from build123d import *

# Parameters (mm, degrees)
SKETCH1_W               = 134.83
SKETCH1_H               = 45.93
SKETCH1_W_2             = 124.83
SKETCH1_H_2             = 35.93
BOSS_EXTRUDE1_DEPTH     = 2.5
BOSS_EXTRUDE2_START     = 2.5
SKETCH1_3_W             = 134.83
SKETCH1_3_H             = 45.93
SKETCH1_3_W_2           = 124.83
SKETCH1_3_H_2           = 35.93
BOSS_EXTRUDE2_DEPTH     = 2.5
SKETCH2_R               = 6.25
SKETCH2_R_2             = 3.25
BOSS_EXTRUDE3_DEPTH     = 5
FILLET1_R               = 10
CUT_EXTRUDE4_DEPTH      = 78.396792246
CUT_EXTRUDE4_DEPTH_BACK = 78.396792246
SKETCH5_W               = 10
SKETCH5_H               = 5
SKETCH6_R               = 1
CUT_EXTRUDE5_DEPTH      = 4
SKETCH7_W               = 7
SKETCH7_H               = 25.4
SKETCH7_W_2             = 8
BOSS_EXTRUDE4_DEPTH     = 7.5
BOSS_EXTRUDE5_START     = -7.5
SKETCH7_4_W             = 8
SKETCH7_4_H             = 25.4
BOSS_EXTRUDE5_DEPTH     = 25.4


with BuildPart() as part:
    # Sketch1 → Boss-Extrude1 (new, symmetric)
    # profile 1 of 2: a face of its own
    with BuildSketch(Plane.XY):
        Rectangle(SKETCH1_W, SKETCH1_H)
        Rectangle(SKETCH1_W_2, SKETCH1_H_2, mode=Mode.SUBTRACT)
    # profile 2 of 2: a face of its own
    with BuildSketch(Plane.XY):
        Rectangle(SKETCH1_W_2, SKETCH1_H_2)
    extrude(amount=BOSS_EXTRUDE1_DEPTH, both=True)

    # Sketch1<3> → Boss-Extrude2 (add, symmetric)
    with BuildSketch(Plane.XY.offset(BOSS_EXTRUDE2_START)):
        Rectangle(SKETCH1_3_W, SKETCH1_3_H)
        Rectangle(SKETCH1_3_W_2, SKETCH1_3_H_2, mode=Mode.SUBTRACT)
    extrude(amount=BOSS_EXTRUDE2_DEPTH, both=True)

    # Sketch2 → Boss-Extrude3 (add)
    # profile 1 of 2: a face of its own
    with BuildSketch(Plane.XZ.offset(22.965)):
        with BuildLine():
            ThreePointArc((6.25, 21.55), (-1.088960505, 15.395597915), (-5.870532806, 23.694608256))
            Line((-5.870532806, 23.694608256), (-12.7, 5))
            Line((-12.7, 5), (12.7, 5))
            Line((12.7, 5), (5.870532806, 23.694608256))
            ThreePointArc((5.870532806, 23.694608256), (6.154402085, 22.638960505), (6.25, 21.55))
        make_face()
    # profile 2 of 2: a face of its own
    with BuildSketch(Plane.XZ.offset(22.965)):
        with Locations((0, 21.55)):
            Circle(SKETCH2_R)
        with Locations(Location((0, 21.55, 0), (0, 0, 270))):
            Circle(SKETCH2_R_2, mode=Mode.SUBTRACT)
    extrude(amount=-BOSS_EXTRUDE3_DEPTH)

    # Fillet1
    fillet1_edges = [part.edges().sort_by_distance(p)[0] for p in [
        (-12.7, -20.465, 5),
        (12.7, -20.465, 5),
    ]]
    fillet(fillet1_edges, radius=FILLET1_R)

    # Sketch5 → Cut-Extrude4 (cut, two sides: drawn at the far end of the back side and taken through both)
    with BuildSketch(Plane(origin=(0, 0, -2.5), x_dir=(-1, 0, 0), z_dir=(0, 0, -1)).offset(-CUT_EXTRUDE4_DEPTH_BACK)):
        with Locations((7, 10.465)):
            Rectangle(SKETCH5_W, SKETCH5_H)
        with Locations((-7, 10.465)):
            Rectangle(SKETCH5_W, SKETCH5_H)
    extrude(amount=CUT_EXTRUDE4_DEPTH + CUT_EXTRUDE4_DEPTH_BACK, mode=Mode.SUBTRACT)

    # Sketch6 → Cut-Extrude5 (cut)
    with BuildSketch(Plane.ZY.offset(2)):
        with Locations((0, 10.465)):
            Circle(SKETCH6_R)
    extrude(amount=-CUT_EXTRUDE5_DEPTH, mode=Mode.SUBTRACT)

    # Sketch7 → Boss-Extrude4 (add)
    with BuildSketch(Plane(origin=(0, 0, -2.5), x_dir=(-1, 0, 0), z_dir=(0, 0, -1))):
        with Locations((-70.915, 0)):
            Rectangle(SKETCH7_W, SKETCH7_H)
        with Locations((-78.415, 0)):
            Rectangle(SKETCH7_W_2, SKETCH7_H)
        with Locations((78.415, 0)):
            Rectangle(SKETCH7_W_2, SKETCH7_H)
        with Locations((70.915, 0)):
            Rectangle(SKETCH7_W, SKETCH7_H)
    extrude(amount=-BOSS_EXTRUDE4_DEPTH)

    # Sketch7<4> → Boss-Extrude5 (add)
    with BuildSketch(Plane(origin=(0, 0, -2.5), x_dir=(-1, 0, 0), z_dir=(0, 0, -1)).offset(BOSS_EXTRUDE5_START)):
        with Locations((-78.415, 0)):
            Rectangle(SKETCH7_4_W, SKETCH7_4_H)
        with Locations((78.415, 0)):
            Rectangle(SKETCH7_4_W, SKETCH7_4_H)
    extrude(amount=-BOSS_EXTRUDE5_DEPTH)


solid = part.part
Work out the finished part from the listing and answer in its coordinate system (mm). A direction names the side the tool comes from. Give positions to 0.01 mm unless a question says otherwise; leave off trailing zeros. Order: outer loops, then holes, each group sorted by start corner. A loop starts at its lowest first (then second) coordinate and runs counter-clockwise, first axis right, second up. Notation, with made-up numbers: M 40.25,-14 L 54.25,-14 A13 ccw 54.25,7 Z; hole C 61,-29.75 d4. An arc over 180 degrees is marked long. Return JSON: item names as keys, results as strings.
Q1. The mould has two halves that part along X. Classify faces 1 (the face through (-77, 12.7, 10)), 2 (the face through (-1, 0, 2.5)), 3 (the face through (8.116, -20.5, 17.547)), 4 (the face through (-67.415, -18, 1)): pulls with the +X half, pulls with the -X half, needs draft (parallel to the pull), parting line crosses it, or undercut.
Answer below:
{"face 1": "needs draft", "face 2": "undercut", "face 3": "pulls with the +X half", "face 4": "pulls with the -X half"}
Q2. Find section C-C, the plane z = 13. Write down the section's boundary in (x, y) (3 decimals), and give its area (3 significant figures).
Answer below:
{"outline": "M -82.415,-12.7 L -74.415,-12.7 L -74.415,12.7 L -82.415,12.7 Z; M -9.777,-22.965 L 9.777,-22.965 L 9.777,-17.965 L -9.777,-17.965 Z; M 74.415,-12.7 L 82.415,-12.7 L 82.415,12.7 L 74.415,12.7 Z", "area": "504 mm^2"}
Q3. Each of these flat-tipped pins is pushed along its axis until it touches: pin 1 (12 mm diameter, centred on x = -74, z = 18.5, fed in from +Y); pin 2 (4 mm diameter, centred on y = -17, z = 1.5, fed in from -X) (3 decimals); pin 3 (6 mm diameter, centred on x = -8.5, z = 24.5, fed in from +Y) (3 decimals). Where does it stop, or does it pass through?
Answer below:
{"pin 1": "stops at y = 12.7", "pin 2": "stops at x = -67.415", "pin 3": "stops at y = -17.965"}
Q4. Find section B-B, the plane y = 15. Write down the section's boundary in (x, z) (3 decimals).
Answer below:
{"outline": "M -67.415,-2.5 L 67.415,-2.5 L 67.415,5 L 62.415,5 L 62.415,2.5 L -62.415,2.5 L -62.415,5 L -67.415,5 Z"}
Q5. Find section A-A, the plane x = 0. Write down the section's boundary in (y, z) (3 decimals), and give its area (3 significant figures).
Answer below:
{"outline": "M -22.965,-2.5 L 22.965,-2.5 L 22.965,5 L 17.965,5 L 17.965,2.5 L -17.965,2.5 L -17.965,18.3 L -22.965,18.3 Z; M -22.965,24.8 L -17.965,24.8 L -17.965,27.8 L -22.965,27.8 Z; hole C 10.465,0 d2", "area": "333 mm^2"}
Q6. Which of the six approach directions +Z, -Z, +X, -X, +Y, -Y give full straight-line access (tool end or side, diameter ignored) to faces 5 (the face through (-74.415, 0, 18)), 6 (the face through (-7, 7.965, 0)), 7 (the face through (0, -17.965, 9)), 8 (the face through (67.415, 18, 1))?
Answer below:
{"face 5": "+Z, +Y, -Y", "face 6": "+Z, -Z", "face 7": "+Z", "face 8": "+Z, -Z, +X, +Y"}
Q7. Find the intervals of material crossed by line 1 along X through (y, z) = (-13, 3) (3 decimals); line 2 along X through (y, z) = (-0.5, 12.5) (3 decimals); line 3 along Z through (x, y) = (-62, -19), in increasing order. Write a range as [from, to].
Answer below:
{"line 1": "x = [-67.415, -62.415], [62.415, 67.415]", "line 2": "x = [-82.415, -74.415], [74.415, 82.415]", "line 3": "z = [-2.5, 5]"}
Q8. Find section D-D, the plane z = 21.55. Write down the section's boundary in (x, y) (3 decimals).
Answer below:
{"outline": "M -82.415,-12.7 L -74.415,-12.7 L -74.415,12.7 L -82.415,12.7 Z; M -6.654,-22.965 L -3.25,-22.965 L -3.25,-17.965 L -6.654,-17.965 Z; M 3.25,-22.965 L 6.654,-22.965 L 6.654,-17.965 L 3.25,-17.965 Z; M 74.415,-12.7 L 82.415,-12.7 L 82.415,12.7 L 74.415,12.7 Z"}
